Part model, mm, in its own coordinate system. Round coordinates to 2 decimals unless told otherwise and drop trailing zeros. Loops run counter-clockwise (first coordinate to the right, second up) from the corner with the lowest first, then second, coordinate; pieces in that order, holes last. Notation, with made-up numbers: M 30.25,69 L 38.25,69 A20 ccw 38.25,87 Z; hole C 18.5,65 d5. An arc over 180 degrees is marked long. Put each result on its own line as item: value. Start each with the question number.
1) Probe line 1 along X through (y, z) = (-50, 0.5); line 2 along X through (y, z) = (-41.5, 0.95); line 3 along Y through (x, z) = (-4.75, 0.35). List the from-to ranges inside material, lowest first.
2) Slice it at B-B on y = 0. Give the cut face in (x, z), then the cut area to 3 significant figures.
3) Slice it at D-D on y = -46.5. Give the cut face in (x, z), then the cut area to 3 significant figures.
4) Slice it at C-C on x = -4.75. Give the cut face in (y, z).
5) Slice it at A-A on z = 0.35. Give the cut face in (x, y), then the cut area to 3 significant figures.
6) Drop flat-ended pins along their axis: pin 1 Ø0.5 at (y, z) = (-21.5, 0.5) entering from +X; pin 2 Ø4 at (x, y) = (0, -39.5) entering from +Z; pin 3 Ø2 at (x, y) = (-4.75, -50) entering from +Z. Give the stop position or say it passes through.
```python
from build123d import *

# Parameters (mm, degrees)
SKETCH2_R           = 1
SKETCH2_R_2         = 0.75
BOSS_EXTRUDE1_DEPTH = 1


with BuildPart() as part:
    # Sketch2 → Boss-Extrude1 (new body)
    with BuildSketch(Plane.XY):
        with BuildLine():
            Line((-6, -4.75), (-6, -50))
            ThreePointArc((-6, -50), (-4.75, -51.25), (-3.5, -50))
            Line((-3.5, -50), (-3.5, -4.75))
            ThreePointArc((-3.5, -4.75), (-2.474873734, -2.275126266), (0, -1.25))
            ThreePointArc((0, -1.25), (1.25, 0), (0, 1.25))
            ThreePointArc((0, 1.25), (-4.242640687, -0.507359313), (-6, -4.75))
        make_face()
        Circle(SKETCH2_R, mode=Mode.SUBTRACT)
        with Locations((-4.75, -50)):
            Circle(SKETCH2_R_2, mode=Mode.SUBTRACT)
    extrude(amount=BOSS_EXTRUDE1_DEPTH)


solid = part.part
```
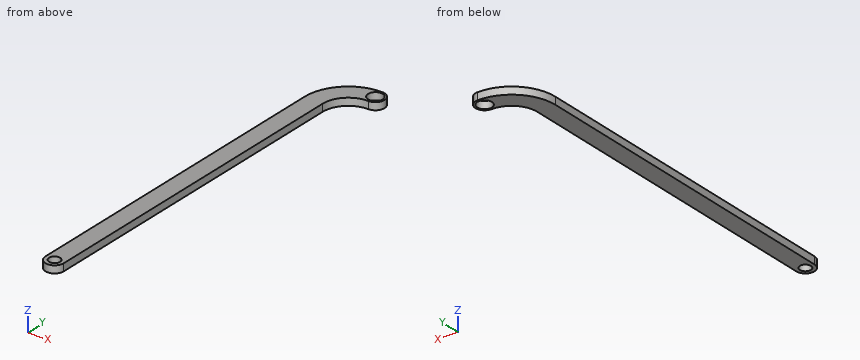
Recorded:
1. line 1: x = -6 to -5.5, -4 to -3.5
1. line 2: x = -6 to -3.5
1. line 3: y = -51.25 to -50.75, -49.25 to -1.08
2. outline: M -3.67,0 L -1,0 L -1,1 L -3.67,1 Z; M 1,0 L 1.25,0 L 1.25,1 L 1,1 Z
2. area: 2.92 mm2
3. outline: M -6,0 L -3.5,0 L -3.5,1 L -6,1 Z
3. area: 2.50 mm2
4. outline: M -51.25,0 L -50.75,0 L -50.75,1 L -51.25,1 Z; M -49.25,0 L -1.08,0 L -1.08,1 L -49.25,1 Z
5. outline: M -6,-50 A1.25 ccw -3.5,-50 L -3.5,-4.75 A3.5 cw 0,-1.25 A1.25 ccw 0,1.25 A6 ccw -6,-4.75 Z; hole C -4.75,-50 d1.5; hole C 0,0 d2
5. area: 132 mm2
6. pin 1: stops at x = -3.5
6. pin 2: passes through
6. pin 3: stops at z = 1
